Work out the finished part from the listing and answer in its coordinate system (mm). A direction names the side the tool comes from. Round coordinates to 2 decimals unless told otherwise and drop trailing zeros. Order: outer loops, then holes, each group sorted by start corner. A loop starts at its lowest first (then second) coordinate and runs counter-clockwise, first axis right, second up. Notation, with made-up numbers: M 29,9.5 L 85,9.5 A31 ccw 85,34.5 Z; hole C 0.25,25.5 d1. An arc over 180 degrees is marked long. Return JSON: item names as keys, results as strings.
from build123d import *

# Parameters (mm, degrees)
SKETCH_R    = 12
SKETCH_R_2  = 3
SKETCH_R_3  = 2.5
PAD_DEPTH   = 10
FILLET_R    = 5
FILLET001_R = 1
FILLET002_R = 10


with BuildPart() as part:
    # Sketch → Pad (new body)
    with BuildSketch(Plane.XY):
        with BuildLine():
            ThreePointArc((-4.031129, -2), (4.5, 0), (-4.031129, 2))
            Line((-4.031129, 2), (-25, 2))
            Line((-25, 45), (-25, 2))
            Line((-25, 45), (55, 45))
            Line((55, 45), (55, -75))
            Line((35, -75), (55, -75))
            Line((35, -115), (35, -75))
            Line((-25, -115), (35, -115))
            Line((-25, -2), (-25, -115))
            Line((-4.031129, -2), (-25, -2))
        make_face()
        with Locations((0, -85)):
            Circle(SKETCH_R, mode=Mode.SUBTRACT)
        with Locations((-10, -52)):
            Circle(SKETCH_R_2, mode=Mode.SUBTRACT)
        with Locations((40, -52)):
            Circle(SKETCH_R_2, mode=Mode.SUBTRACT)
        with Locations((40, 22)):
            Circle(SKETCH_R_2, mode=Mode.SUBTRACT)
        with Locations((-10, 22)):
            Circle(SKETCH_R_2, mode=Mode.SUBTRACT)
        with Locations((25, -80)):
            Circle(SKETCH_R_3, mode=Mode.SUBTRACT)
        with Locations((-18, -80)):
            Circle(SKETCH_R_3, mode=Mode.SUBTRACT)
    extrude(amount=PAD_DEPTH)

    # Fillet
    fillet_edges = [part.edges().sort_by_distance(p)[0] for p in [
        (35, -75, 5),
    ]]
    fillet(fillet_edges, radius=FILLET_R)

    # Fillet001
    fillet001_edges = [part.edges().sort_by_distance(p)[0] for p in [
        (55, -75, 5),
        (55, 45, 5),
        (-25, 2, 5),
        (-25, -2, 5),
        (-25, 45, 5),
    ]]
    fillet(fillet001_edges, radius=FILLET001_R)

    # Fillet002
    fillet002_edges = [part.edges().sort_by_distance(p)[0] for p in [
        (-25, -115, 5),
        (35, -115, 5),
    ]]
    fillet(fillet002_edges, radius=FILLET002_R)


solid = part.part
Item 1: Consider line 1 along Y through (x, z) = (0, 1.5); line 2 along Y through (x, z) = (-20, 4.5); line 3 along Y through (x, z) = (-10, 7.5). Determine where each line is inside the solid, lowest interval first. Write a range as [from, to].
Output:
{"line 1": "y = [-115, -97], [-73, -4.5], [4.5, 45]", "line 2": "y = [-113.66, -81.5], [-78.5, -2], [2, 45]", "line 3": "y = [-115, -91.63], [-78.37, -55], [-49, -2], [2, 19], [25, 45]"}
Item 2: The mould has two halves that part along Y. Classify faces 3 (the flat face through (-14, -2, 5)), 4 (the flat face through (-25, 24, 5)), 5 (the cylindrical face through (-21.99, -112.15, 5.07)), 6 (the flat face through (-14, 2, 5)): pulls with the +Y half, pulls with the -Y half, needs draft (parallel to the pull), parting line crosses it, or undercut.
Output:
{"face 3": "undercut", "face 4": "needs draft", "face 5": "pulls with the -Y half", "face 6": "undercut"}
Item 3: Find section C-C (y = -52). Determine the outline of the cut face in (x, z).
Output:
{"outline": "M -25,0 L -13,0 L -13,10 L -25,10 Z; M -7,0 L 37,0 L 37,10 L -7,10 Z; M 43,0 L 55,0 L 55,10 L 43,10 Z"}
Item 4: Find section A-A (z = 8). Determine the outline of the cut face in (x, y).
Output:
{"outline": "M -25,-105 A10 ccw -15,-115 L 25,-115 A10 ccw 35,-105 L 35,-80 A5 cw 40,-75 L 54,-75 A1 ccw 55,-74 L 55,44 A1 ccw 54,45 L -24,45 A1 ccw -25,44 L -25,3 A1 ccw -24,2 L -4.03,2 A4.5 cw long -4.03,-2 L -24,-2 A1 ccw -25,-3 Z; hole C -18,-80 d5; hole C -10,-52 d6; hole C -10,22 d6; hole C 0,-85 d24; hole C 25,-80 d5; hole C 40,-52 d6; hole C 40,22 d6"}
Item 5: Which of the six approach directions +Z, -Z, +X, -X, +Y, -Y give full straight-line access (tool end or side, diameter ignored) to faces 1 (the cylindrical face through (-10, -49, 5)), 2 (the flat face through (47, -75, 5))?
Output:
{"face 1": "+Z, -Z", "face 2": "+Z, -Z, +X, -Y"}
Item 6: Each of these flat-tipped pins is pushed along its axis until it touches: pin 1 (3 mm diameter, centred on x = 49, z = 5.5, fed in from -Y); pin 2 (3 mm diameter, centred on x = -17, z = 6, fed in from -Y); pin 3 (5 mm diameter, centred on x = 39.5, z = 6.5, fed in from -Y). Where does it stop, or does it pass through?
Output:
{"pin 1": "stops at y = -75", "pin 2": "stops at y = -114.99", "pin 3": "stops at y = -76"}
Item 7: Find section B-B (y = -85). Determine the outline of the cut face in (x, z), plus the area to 3 significant figures.
Output:
{"outline": "M -25,0 L -12,0 L -12,10 L -25,10 Z; M 12,0 L 35,0 L 35,10 L 12,10 Z", "area": "360 mm^2"}
Item 8: Find section D-D (x = -10). Determine the outline of the cut face in (y, z).
Output:
{"outline": "M -115,0 L -91.63,0 L -91.63,10 L -115,10 Z; M -78.37,0 L -55,0 L -55,10 L -78.37,10 Z; M -49,0 L -2,0 L -2,10 L -49,10 Z; M 2,0 L 19,0 L 19,10 L 2,10 Z; M 25,0 L 45,0 L 45,10 L 25,10 Z"}
